Autodesk Inventor part; units mm, degrees
ref_plane "YZ Plane" through (0, 0, 0) normal (1, 0, 0) x (0, 1, 0)
ref_plane "XZ Plane" through (0, 0, 0) normal (0, 1, 0) x (-1, 0, 0)
ref_plane "XY Plane" through (0, 0, 0) normal (0, 0, 1) x (1, 0, 0)
sketch "Szkic1" plane through (0, 0, 0) normal (0, 1, 0) x (-1, 0, 0)
  circle A0 centre (0, 0) radius 5
  line L0 (7.5, 0) -> (5, 0)
  line L1 (7.5, -4.3301) -> (0, -8.6603)
  line L2 (0, -8.6603) -> (-7.5, -4.3301)
  line L3 (-7.5, -4.3301) -> (-7.5, 4.3301)
  line L4 (-7.5, 4.3301) -> (0, 8.6603)
  line L5 (0, 8.6603) -> (7.5, 4.3301)
  line L6 (7.5, 4.3301) -> (7.5, -4.3301)
extrude "Wyciągnięcie proste1" add sketch "Szkic1" along normal blind 10
thread "Gwint1"
properties part number "Nakrętka trapezowa 10x17"
For this review, take the finished solid that the model builds, in its own axes (mm). Give positions to 0.01 mm unless a question says otherwise; leave off trailing zeros. Write each loop counter-clockwise with the first axis right and the second up, starting at its lowest first coordinate (ties: lowest second). Pieces come first, ordered by that corner, then holes. Notation, with made-up numbers: M 67.25,38.5 L 75.25,38.5 A7 cw 75.25,43.5 Z; hole C 25,41 d4. An arc over 180 degrees is marked long. Answer as a JSON object with one key per item and string values. Group by question number.
Item 1: Consider section B-B on x = 0.5. Write out the cut boundary in (y, z), plus the area to 3 significant figures.
Item 2: Consider section D-D on z = 5.5. Write out the cut boundary in (x, y), plus the area to 3 significant figures.
Item 3: For probe 1 along Z at (x, y) = (-2.5, 1.25); probe 2 along X at (y, z) = (4.75, -3); probe 3 along X at (y, z) = (1.5, -0.25), list the stretches that pass through material, from the lowest coordinate up. Write a range as [from, to].
Item 4: Draft analysis for pull direction X (two halves, no side actions). For faces 1 (the flat face through (7.5, 5, 0)), 2 (the flat face through (-7.5, 5, 0)), 3 (the cylindrical face through (1.08, 4.93, 4.88)), 4 (the flat face through (5, 0, -2)), state which applies: +X half, -X half, draft (parallel to the pull), parting line (faces both ways), or undercut.
Item 5: For pin 1 Ø3 at (x, y) = (2, 1) entering from -Z; pin 2 Ø4 at (x, z) = (-2.5, -1.5) entering from +Y; pin 3 Ø6 at (y, z) = (1.5, 4.5) entering from -X; pin 4 Ø2 at (x, y) = (-2.5, 5) entering from -Z, all flat-tipped, find the tip position at first contact; note any pin that passes through.
Item 6: Consider section C-C on y = 2.25. Write out the cut boundary in (x, z), plus the area to 3 significant figures.
Item 7: Consider section A-A on z = 3. Write out the cut boundary in (x, y), plus the area to 3 significant figures.
Check result:
{
 "1": {"outline": "M 0,-8.37 L 10,-8.37 L 10,-4.97 L 0,-4.97 Z; M 0,4.97 L 10,4.97 L 10,8.37 L 0,8.37 Z", "area": "67.9 mm^2"},
 "2": {"outline": "M -5.47,0 L 5.47,0 L 5.47,10 L -5.47,10 Z", "area": "109 mm^2"},
 "3": {"probe 1": "z = [-7.22, -4.33], [4.33, 7.22]", "probe 2": "x = [-7.5, -4], [4, 7.5]", "probe 3": "x = [-7.5, -4.99], [4.99, 7.5]"},
 "4": {"face 1": "+X half", "face 2": "-X half", "face 3": "undercut", "face 4": "draft"},
 "5": {"pin 1": "stops at z = -8.37", "pin 2": "passes through", "pin 3": "stops at x = -7.5", "pin 4": "stops at z = -7.79"},
 "6": {"outline": "M -7.5,-4.33 L 0,-8.66 L 7.5,-4.33 L 7.5,4.33 L 0,8.66 L -7.5,4.33 Z; hole C 0,0 d10", "area": "116 mm^2"},
 "7": {"outline": "M -7.5,0 L -4,0 L -4,10 L -7.5,10 Z; M 4,0 L 7.5,0 L 7.5,10 L 4,10 Z", "area": "70.0 mm^2"}
}
